Geometry: final body of the model. Coordinates: model frame, mm. Give positions to 0.01 mm unless a question says otherwise; leave off trailing zeros. Write each loop counter-clockwise with the first axis right and the second up, starting at its lowest first coordinate (ties: lowest second). Pieces come first, ordered by that corner, then holes.
Q1. Pin query (flat end, axial travel): pin 1 Ø3 at (x, z) = (15, 3) entering from -Y. Return the tip coordinate at first contact, or that it passes through.
Q2. Section B-B (z = 31). Return the cut outline in (x, y) (3 decimals).
Q3. Section A-A (x = 15). Return the cut outline in (y, z) (3 decimals).
Q4. Line query: line 1 (X direction, y = 1.4, z = 3); line 2 (X direction, y = 0.95, z = 31) (3 decimals); line 3 (Z direction, x = 2.5, y = 1.75) (3 decimals). Output: solid intervals per line, ascending.
Q5. Mould query, pull axis Z, two halves, no side actions, for faces 1 (the flat face through (25, 2, 0)), 2 (the flat face through (50, 2, 28)), 3 (the cylindrical face through (1.839, 1.565, 32.593)). Classes: +Z half, -Z half, draft (parallel to the pull), parting line (faces both ways), or undercut.
Q6. Section C-C (x = 2.5). Return the cut outline in (y, z) (3 decimals), plus the area to 3 significant figures.
from build123d import *

# Parameters (mm, degrees)
SKETCH1_W               = 50
SKETCH1_H               = 56
SKETCH1_R               = 1.1
BOSS_EXTRUDE1_DEPTH     = 3.175
FILLET1_R               = 1
M3X0_5_TAPPED_HOLE1_D   = 2.5
CUT_EXTRUDE1_DEPTH      = 76.140406074
CUT_EXTRUDE1_DEPTH_BACK = 76.140406074
SKETCH3_R               = 1.725


with BuildPart() as part:
    # Sketch1 → Boss-Extrude1 (new body)
    with BuildSketch(Plane(origin=(0, 0, 0), x_dir=(1, 0, 0), z_dir=(0, 1, 0))):
        with Locations((25, -28)):
            Rectangle(SKETCH1_W, SKETCH1_H)
        with Locations(Location((15, -3, 0), (0, 0, 270))):
            Circle(SKETCH1_R, mode=Mode.SUBTRACT)
        with Locations(Location((35, -3, 0), (0, 0, 270))):
            Circle(SKETCH1_R, mode=Mode.SUBTRACT)
    extrude(amount=BOSS_EXTRUDE1_DEPTH)

    # Fillet1
    fillet1_edges = [part.edges().sort_by_distance(p)[0] for p in [
        (0, 1.5875, 0),
        (50, 1.5875, 0),
        (50, 1.5875, 56),
        (0, 1.5875, 56),
    ]]
    fillet(fillet1_edges, radius=FILLET1_R)

    # M3x0.5 Tapped Hole1 (through all)
    with Locations(Plane(origin=(15, 3.175, 3), x_dir=(0, 0, 1), z_dir=(0, 1, 0))):
        with Locations((0, 0), (0, 20)):
            Hole(M3X0_5_TAPPED_HOLE1_D / 2)

    # Sketch3 → Cut-Extrude1 (cut, two sides: drawn at the far end of the back side and taken through both)
    with BuildSketch(Plane(origin=(0, 3.175, 0), x_dir=(1, 0, 0), z_dir=(0, 1, 0)).offset(-CUT_EXTRUDE1_DEPTH_BACK)):
        with Locations(Location((2.5, -31, 0), (0, 0, 270))):
            Circle(SKETCH3_R)
        with Locations(Location((47.5, -31, 0), (0, 0, 270))):
            Circle(SKETCH3_R)
    extrude(amount=CUT_EXTRUDE1_DEPTH + CUT_EXTRUDE1_DEPTH_BACK, mode=Mode.SUBTRACT)


solid = part.part
Computed:
1. pin 1: stops at y = 0
2. outline: (0, 0) - (0.775, 0) - (0.775, 3.175) - (0, 3.175) - close; (4.225, 0) - (45.775, 0) - (45.775, 3.175) - (4.225, 3.175) - close; (49.225, 0) - (50, 0) - (50, 3.175) - (49.225, 3.175) - close
3. outline: (0, 0) - (3.175, 0) - (3.175, 1.75) - (0, 1.75) - close; (0, 4.25) - (3.175, 4.25) - (3.175, 56) - (0, 56) - close
4. line 1: x = 0 to 13.75, 16.25 to 33.75, 36.25 to 50
4. line 2: x = 0 to 0.775, 4.225 to 45.775, 49.225 to 50
4. line 3: z = 0 to 29.275, 32.725 to 56
5. face 1: -Z half
5. face 2: draft
5. face 3: undercut
6. outline: (0, 0) - (3.175, 0) - (3.175, 29.275) - (0, 29.275) - close; (0, 32.725) - (3.175, 32.725) - (3.175, 56) - (0, 56) - close
6. area: 167 mm2
